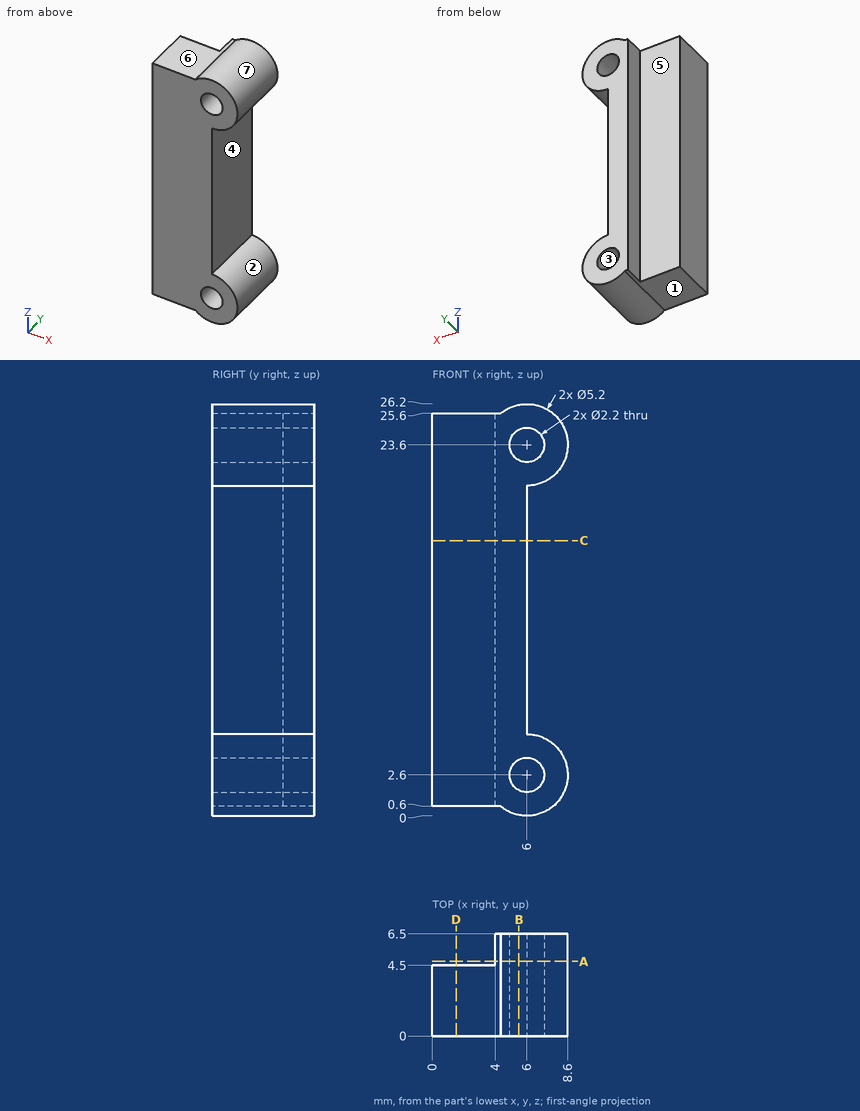
Input: dimensioned drawing with shaded views. Units: mm. Origin: part minimum x, y, z. A direction names the side the tool comes from. Round coordinates to 2 decimals unless told otherwise and drop trailing zeros. Order: outer loops, then holes, each group sorted by start corner. A loop starts at its lowest first (then second) coordinate and runs counter-clockwise, first axis right, second up. Notation, with made-up numbers: (67, 73) -> (106, 73) arc R23 ccw to (106, 99) -> close; hole circle Ø3 at (-15, 78). An arc over 180 degrees is marked (long way). Put each result on its own line as item: value. Start each with the question number.
Q1. First-contact query: pin 1 (2 mm diameter, centred on x = 6, z = 2.6, fed in from -Y); pin 2 (3 mm diameter, centred on x = 2, z = 15.5, fed in from +Y); pin 3 (1 mm diameter, centred on x = 3.5, y = 2, fed in from +Z); pin 4 (0.6 mm diameter, centred on y = 5, z = 17, fed in from -X). Flat tips, straight axial feed; report the tip coordinate or a pass-through.
Q2. Section D-D on x = 1.5. Return the cut outline in (y, z).
Q3. Section B-B on x = 5.5. Return the cut outline in (y, z).
Q4. Section C-C on z = 17.5. Return the cut outline in (x, y).
Q5. Line query: probe 1 along X at (y, z) = (6, 9); probe 2 along X at (y, z) = (3, 15.25); probe 3 along Y at (x, z) = (3.5, 7.5). Output: solid intervals per line, ascending.
Q6. Reachability of the marked faces 5, 6 and 7 from +Z, -Z, +X, -X, +Y, -Y: full face, straight path, thin tool, end or side. Return the list, or none.
Q7. Section A-A on y = 4.75. Return the cut outline in (x, z), and give its area (3 significant figures).
Q8. Pull-direction query (X, two-part tool) for the marked faces 1, 2, 3 and 4; classes: +X half, -X half, draft (parallel to the pull), parting line (faces both ways), or undercut.
Ans:
1. pin 1: passes through
1. pin 2: stops at y = 4.5
1. pin 3: stops at z = 25.6
1. pin 4: stops at x = 4
2. outline: (0, 0.6) -> (4.5, 0.6) -> (4.5, 25.6) -> (0, 25.6) -> close
3. outline: (0, 0.05) -> (6.5, 0.05) -> (6.5, 1.62) -> (0, 1.62) -> close; (0, 3.58) -> (6.5, 3.58) -> (6.5, 22.62) -> (0, 22.62) -> close; (0, 24.58) -> (6.5, 24.58) -> (6.5, 26.15) -> (0, 26.15) -> close
4. outline: (0, 0) -> (6, 0) -> (6, 6.5) -> (4, 6.5) -> (4, 4.5) -> (0, 4.5) -> close
5. probe 1: x = 4 to 6
5. probe 2: x = 0 to 6
5. probe 3: y = 0 to 4.5
6. face 5: +Z, -Z, -X, +Y
6. face 6: +Z, -X, +Y, -Y
6. face 7: +Y, -Y
7. outline: (4, 0.6) -> (4.34, 0.6) arc R2.6 ccw (long way) to (6, 5.2) -> (6, 21) arc R2.6 ccw (long way) to (4.34, 25.6) -> (4, 25.6) -> close; hole circle Ø2.2 at (6, 2.6); hole circle Ø2.2 at (6, 23.6)
7. area: 65.0 mm2
8. face 1: draft
8. face 2: parting line
8. face 3: undercut
8. face 4: +X half
